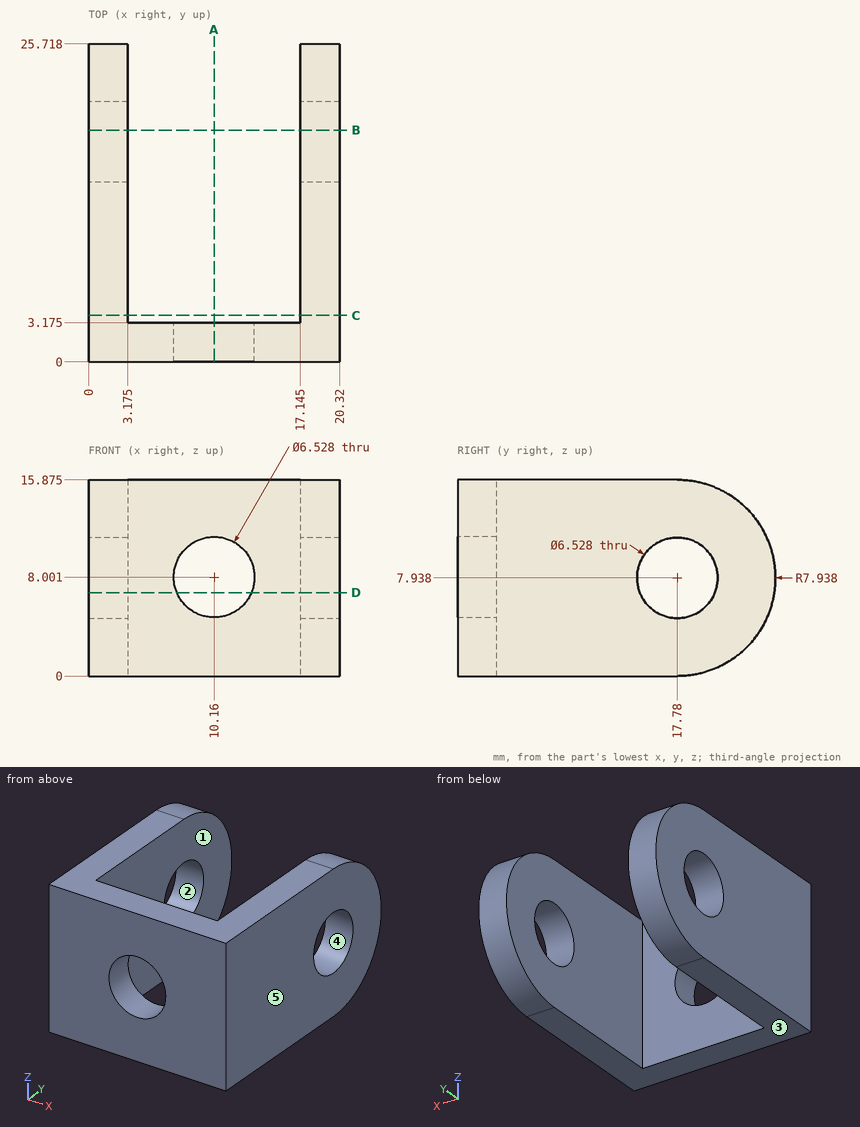
Input: dimensioned drawing with shaded views. Units: mm. Origin: part minimum x, y, z. A direction names the side the tool comes from. Round coordinates to 2 decimals unless told otherwise and drop trailing zeros. Loops run counter-clockwise (first coordinate to the right, second up) from the corner with the lowest first, then second, coordinate; pieces in that order, holes last. Notation, with made-up numbers: (87.5, 35) -> (146.5, 35) arc R10 ccw to (146.5, 45) -> close; hole circle Ø2 at (38, 34.5). An arc over 180 degrees is marked (long way). Use one line per item in the form item = value. Start each with the question number.
1) First-contact query: P1, Ø8, axis at y = 16.5, z = 8, coming from the -X side; P2, Ø1.5, axis at x = 10, z = 9.5, coming from the -Y side; P3, Ø2, axis at x = 17, z = 12.5, coming from the +Y side. Flat tips, straight axial feed; report the tip coordinate or a pass-through.
2) Access query for the marked faces 1 and 2. Directions: +Z, -Z, +X, -X, +Y, -Y. A direction counts if a zero-diameter tool reaches every point of the face in a straight line with its end or side. Return the directions, or none.
3) Section C-C on y = 3.75. Output: boundary loops of the cut face in (x, z) (1 decimal), then the cut area to 3 significant figures.
4) Section A-A on x = 10.16. Output: boundary loops of the cut face in (y, z) (1 decimal).
5) Section D-D on z = 6.75. Output: boundary loops of the cut face in (x, y) (1 decimal).
6) Draft query along Z for the marked faces 3, 4 and 5. Return one class per face: released by +Z, released by -Z, zero draft, split by the parting line, or undercut.
7) Section B-B on y = 18.75. Output: boundary loops of the cut face in (x, z) (1 decimal).
8) Line query: L1, parallel to X at y = 7.25, z = 15 (1 decimal); L2, parallel to Y at x = 1, z = 7.75 (1 decimal); L3, parallel to Y at x = 14.5, z = 2.75 (1 decimal). Output: solid intervals per line, ascending.
Response:
q1.P1 = 0
q1.P2 = through
q1.P3 = 24.87
q2.face_1 = +Z, -Z, +Y
q2.face_2 = +X, -X
q3.outline = (0, 0) -> (3.2, 0) -> (3.2, 15.9) -> (0, 15.9) -> close; (17.1, 0) -> (20.3, 0) -> (20.3, 15.9) -> (17.1, 15.9) -> close
q3.area = 101 mm^2
q4.outline = (0, 0) -> (3.2, 0) -> (3.2, 4.7) -> (0, 4.7) -> close; (0, 11.3) -> (3.2, 11.3) -> (3.2, 15.9) -> (0, 15.9) -> close
q5.outline = (0, 0) -> (7.1, 0) -> (7.1, 3.2) -> (3.2, 3.2) -> (3.2, 14.7) -> (0, 14.7) -> close; (0, 20.8) -> (3.2, 20.8) -> (3.2, 25.6) -> (0, 25.6) -> close; (13.2, 0) -> (20.3, 0) -> (20.3, 14.7) -> (17.1, 14.7) -> (17.1, 3.2) -> (13.2, 3.2) -> close; (17.1, 20.8) -> (20.3, 20.8) -> (20.3, 25.6) -> (17.1, 25.6) -> close
q6.face_3 = released by -Z
q6.face_4 = undercut
q6.face_5 = zero draft
q7.outline = (0, 0.1) -> (3.2, 0.1) -> (3.2, 4.8) -> (0, 4.8) -> close; (0, 11.1) -> (3.2, 11.1) -> (3.2, 15.8) -> (0, 15.8) -> close; (17.1, 0.1) -> (20.3, 0.1) -> (20.3, 4.8) -> (17.1, 4.8) -> close; (17.1, 11.1) -> (20.3, 11.1) -> (20.3, 15.8) -> (17.1, 15.8) -> close
q8.L1 = 0 to 3.2, 17.1 to 20.3
q8.L2 = 0 to 14.5, 21 to 25.7
q8.L3 = 0 to 3.2
